```python
from build123d import *

# Parameters (mm, degrees)
BOX_W           = 25
BOX_H           = 10
BOX_DEPTH       = 10
SKETCH_W        = 4
SKETCH_H        = 10
PAD_DEPTH       = 8
PAD_DEPTH_BACK  = 18
SKETCH001_R     = 1.5
POCKET_DEPTH    = 25.001
SKETCH002_R     = 3
POCKET001_DEPTH = 20
SKETCH003_R     = 1.5
POCKET002_DEPTH = 8.001
SKETCH004_R     = 2.6
POCKET003_DEPTH = 2
FILLET_R        = 1


with BuildPart() as part:
    # Box → Box (new body)
    with BuildSketch(Plane.XY):
        with Locations((12.5, 5)):
            Rectangle(BOX_W, BOX_H)
    extrude(amount=BOX_DEPTH)

    # Sketch → Pad (new body, two sides)
    with BuildSketch(Plane.XZ) as pad_sk:
        with Locations((6, 5)):
            Rectangle(SKETCH_W, SKETCH_H)
    extrude(amount=PAD_DEPTH)
    extrude(pad_sk.sketch, amount=-PAD_DEPTH_BACK)

    # Sketch001 → Pocket (cut, through all)
    with BuildSketch(Plane.YZ.offset(25)):
        with Locations((5, 5)):
            Circle(SKETCH001_R)
    extrude(amount=-POCKET_DEPTH, mode=Mode.SUBTRACT)

    # Sketch002 → Pocket001 (cut)
    with BuildSketch(Plane.YZ.offset(25)):
        with Locations((5, 5)):
            Circle(SKETCH002_R)
    extrude(amount=-POCKET001_DEPTH, mode=Mode.SUBTRACT)

    # Sketch003 → Pocket002 (cut, through all)
    with BuildSketch(Plane.YZ.offset(8)):
        with Locations((-4, 5)):
            Circle(SKETCH003_R)
        with Locations((14, 5)):
            Circle(SKETCH003_R)
    extrude(amount=-POCKET002_DEPTH, mode=Mode.SUBTRACT)

    # Sketch004 → Pocket003 (cut)
    with BuildSketch(Plane.YZ.offset(8)):
        with Locations((-4, 5)):
            Circle(SKETCH004_R)
        with Locations((14, 5)):
            Circle(SKETCH004_R)
    extrude(amount=-POCKET003_DEPTH, mode=Mode.SUBTRACT)

    # Fillet
    fillet_edges = [part.edges().sort_by_distance(p)[0] for p in [
        (25, 5, 10),
        (25, 0, 5),
        (25, 5, 0),
        (25, 10, 5),
    ]]
    fillet(fillet_edges, radius=FILLET_R)


solid = part.part
```
Can you work these out from the model? Positions are in its coordinate system, mm. A direction names the side the tool comes from. Round coordinates to 2 decimals unless told otherwise and drop trailing zeros. Loops run counter-clockwise (first coordinate to the right, second up) from the corner with the lowest first, then second, coordinate; pieces in that order, holes last.
Item 1: Please list where these lines run through material, in increasing order: L1, parallel to Z at x = 4.9, y = 14; L2, parallel to Z at x = 6.75, y = 14.
Item 2: Suppose I cut it at A-A, the plane y = 5. Write out the boundary of the cut face in (x, z), then the cut area to 3 significant figures.
Item 3: Suppose I cut it at B-B, the plane x = 7.25. Write out the boundary of the cut face in (y, z), then the cut area to 3 significant figures.
Item 4: Which directions (+Z, -Z, +X, -X, +Y, -Y) give clear straight access to the entire face, cutting with the end or side of a thin tool? Please do faces 5 (the flat face through (12, 5, 0)), 6 (the flat face through (2, 10, 5)), 7 (the flat face through (4, -2, 5)), 8 (the flat face through (16, 0, 5)), 9 (the cylindrical face through (7.01, -1.52, 5.78)).
Item 5: Suppose I cut it at C-C, the plane z = 8.5. Write out the boundary of the cut face in (x, y), then the cut area to 3 significant figures.
Item 6: Will these pins go through, and if not, where does the flat tip stop? pin 1 Ø5.5 at (y, z) = (13, 5) entering from +X; pin 2 Ø4 at (x, z) = (11, 2) entering from -Y; pin 3 Ø3.5 at (y, z) = (14, 5) entering from +X.
Item 7: Suppose I cut it at D-D, the plane x = 10. Write out the boundary of the cut face in (y, z).
Item 8: If we mould it in two halves opening along Y, with no side actions, what happens to faces 1 (the cylindrical face through (24.699, 5.07, 9.715)), 2 (the flat face through (6, -8, 5)), 3 (the cylindrical face through (7.01, 16.48, 5.78)), 4 (the cylindrical face through (24.715, 9.699, 5.07))? For each: +Y half, -Y half, draft (parallel to the pull), parting line (faces both ways), or undercut.
Reported:
1. L1: z = 0 to 3.5, 6.5 to 10
1. L2: z = 0 to 2.4, 7.6 to 10
2. outline: (0, 0) - (24, 0) arc R1 ccw to (25, 1) - (25, 2) - (5, 2) - (5, 3.5) - (0, 3.5) - close; (0, 6.5) - (5, 6.5) - (5, 8) - (25, 8) - (25, 9) arc R1 ccw to (24, 10) - (0, 10) - close
2. area: 115 mm2
3. outline: (-8, 0) - (18, 0) - (18, 10) - (-8, 10) - close; hole circle Ø5.2 at (-4, 5); hole circle Ø6 at (5, 5); hole circle Ø5.2 at (14, 5)
3. area: 189 mm2
4. face 5: -Z, +X, -X, +Y, -Y
4. face 6: +Z, -Z, -X, +Y
4. face 7: +Z, -Z, -X, -Y
4. face 8: +Z, -Z, +X, -Y
4. face 9: +X
5. outline: (0, 0) - (4, 0) - (4, -8) - (8, -8) - (8, 0) - (24, 0) arc R1 ccw to (25, 1) - (25, 9) arc R1 ccw to (24, 10) - (8, 10) - (8, 18) - (4, 18) - (4, 10) - (0, 10) - close
5. area: 314 mm2
6. pin 1: stops at x = 8
6. pin 2: stops at y = 0
6. pin 3: stops at x = 6
7. outline: (0, 0) - (10, 0) - (10, 10) - (0, 10) - close; hole circle Ø6 at (5, 5)
8. face 1: draft
8. face 2: -Y half
8. face 3: undercut
8. face 4: +Y half
